Input: part model. Units: mm. Frame: model coordinates. A direction names the side the tool comes from. Give positions to 0.01 mm unless a question says otherwise; leave off trailing zeros. Write each loop counter-clockwise with the first axis right and the second up, starting at its lowest first coordinate (ties: lowest second). Pieces come first, ordered by that corner, then holes.
```python
from build123d import *

# Parameters (mm, degrees)
SKETCH1_W           = 88.9
SKETCH1_H           = 7.3406
BOSS_EXTRUDE1_DEPTH = 6.35
SKETCH2_W           = 88.9
SKETCH2_H           = 3.175
CUT_EXTRUDE2_DEPTH  = 4.7625
CUT_EXTRUDE3_DEPTH  = 7.3406
SKETCH5_R           = 1.025
CUT_EXTRUDE4_DEPTH  = 1.5875


with BuildPart() as part:
    # Sketch1 → Boss-Extrude1 (new body)
    with BuildSketch(Plane(origin=(0, 0, 0), x_dir=(0, 0, -1), z_dir=(1, 0, 0))):
        with Locations((44.45, 3.6703)):
            Rectangle(SKETCH1_W, SKETCH1_H)
    extrude(amount=BOSS_EXTRUDE1_DEPTH)

    # Sketch2 → Cut-Extrude2 (cut)
    with BuildSketch(Plane(origin=(6.35, 0, 0), x_dir=(0, 0, -1), z_dir=(1, 0, 0))):
        with Locations((44.45, 3.6703)):
            Rectangle(SKETCH2_W, SKETCH2_H)
    extrude(amount=-CUT_EXTRUDE2_DEPTH, mode=Mode.SUBTRACT)

    # Sketch4 → Cut-Extrude3 (cut)
    with BuildSketch(Plane.XZ):
        Polygon((0, 0), (6.35, -10.998522628), (6.35, 0), align=None)
        Polygon((6.35, -77.901477372), (6.35, -88.9), (0, -88.9), align=None)
    extrude(amount=-CUT_EXTRUDE3_DEPTH, mode=Mode.SUBTRACT)

    # Sketch5 → Cut-Extrude4 (cut)
    with BuildSketch(Plane.ZY):
        with Locations((-76.2, 3.6703)):
            Circle(SKETCH5_R)
        with Locations((-44.45, 3.6703)):
            Circle(SKETCH5_R)
        with Locations(Location((-12.7, 3.6703, 0), (0, 0, 180))):
            Circle(SKETCH5_R)
    extrude(amount=-CUT_EXTRUDE4_DEPTH, mode=Mode.SUBTRACT)


solid = part.part
```
Item 1: Section A-A (z = -44.45). Return loops of the section in (x, y).
Item 2: Set-up query: faces 4 (the cylindrical face through (0.783, 3.715, -77.224)), 5 (the flat face through (4, 5.258, -44)). Return all of +Z, -Z, +X, -X, +Y, -Y with unobstructed straight access to the full face (end or side cutting, diameter ignored); none if empty.
Item 3: Section C-C (z = -15.5). Return loops of the section in (x, y), and give its area (3 significant figures).
Item 4: Section D-D (y = 6.25). Return loops of the section in (x, z).
Item 5: Section B-B (x = 5.25). Return loops of the section in (y, z).
Item 6: Pin query (flat end, axial travel): pin 1 (1 mm diameter, centred on y = 3.5, z = -41.5, fed in from +X). Return the tip coordinate at first contact, or that it passes through.
Item 7: Ray query, line 1 (Y direction, x = 3.75, z = -80); line 2 (Y direction, x = 1.05, z = -12.7); line 3 (Z direction, x = 1, y = 2.75). Return the intervals inside material, ascending.
Item 8: Mould query, pull axis Z, two halves, no side actions, for faces 1 (the flat face through (6.35, 1, -44)), 2 (the flat face through (2.425, 1.172, -84.7)), 3 (the cylindrical face through (0.783, 3.978, -43.472)). Classes: +Z half, -Z half, draft (parallel to the pull), parting line (faces both ways), or undercut.
Solved:
1. outline: (0, 0) - (6.35, 0) - (6.35, 2.08) - (1.59, 2.08) - (1.59, 2.65) - (0, 2.65) - close; (0, 4.7) - (1.59, 4.7) - (1.59, 5.26) - (6.35, 5.26) - (6.35, 7.34) - (0, 7.34) - close
2. face 4: +X, -X
2. face 5: +Z, -Z, +X
3. outline: (0, 0) - (6.35, 0) - (6.35, 2.08) - (1.59, 2.08) - (1.59, 5.26) - (6.35, 5.26) - (6.35, 7.34) - (0, 7.34) - close
3. area: 31.5 mm2
4. outline: (0, -88.9) - (6.35, -77.9) - (6.35, -11) - (0, 0) - close
5. outline: (0, -79.81) - (2.08, -79.81) - (2.08, -9.09) - (0, -9.09) - close; (5.26, -79.81) - (7.34, -79.81) - (7.34, -9.09) - (5.26, -9.09) - close
6. pin 1: stops at x = 1.59
7. line 1: y = 0 to 2.08, 5.26 to 7.34
7. line 2: y = 0 to 2.65, 4.7 to 7.34
7. line 3: z = -87.17 to -76.65, -75.75 to -44.9, -44 to -13.15, -12.25 to -1.73
8. face 1: draft
8. face 2: -Z half
8. face 3: undercut
